```python
from build123d import *
from build123d.topology import SkipClean

# Parameters (mm, degrees)
SKETCH1_R           = 9.525
BOSS_EXTRUDE1_DEPTH = 250
BOSS_EXTRUDE2_DEPTH = 1.5875
CUT_EXTRUDE1_REACH  = 503.261
SKETCH3_R           = 4
SKETCH4_R           = 9.525
BOSS_EXTRUDE3_DEPTH = 50


with BuildPart() as part:
    # Sketch1 → Boss-Extrude1 (new, symmetric)
    with BuildSketch(Plane.XY):
        Circle(SKETCH1_R)
    extrude(amount=BOSS_EXTRUDE1_DEPTH, both=True)

    # Sketch2 → Boss-Extrude2 (add, symmetric)
    with SkipClean():  # the faces are left unmerged after this step: merging them gives an invalid solid
        with BuildSketch(Plane(origin=(0, 0, -250), x_dir=(-1, 0, 0), z_dir=(0, 0, -1))):
            with BuildLine():
                Line((-9.32999835, 1.91748684), (-18.518650577, -42.792134274))
                ThreePointArc((-18.518650577, -42.792134274), (-17.291604236, -47.791622716), (-12.641486262, -50))
                Line((-12.641486262, -50), (12.641486262, -50))
                ThreePointArc((12.641486262, -50), (17.291604236, -47.791622716), (18.518650577, -42.792134274))
                Line((18.518650577, -42.792134274), (9.32999835, 1.91748684))
                ThreePointArc((9.32999835, 1.91748684), (0, 9.525), (-9.32999835, 1.91748684))
            make_face()
        extrude(amount=BOSS_EXTRUDE2_DEPTH, both=True)
    add(part.part.scale(1), mode=Mode.REPLACE)  # the faces are merged on a copy

    # Sketch3 → Cut-Extrude1 (cut, up to next)
    with BuildSketch(Plane.XY.offset(-248.4125), mode=Mode.PRIVATE) as cut_extrude1_sk1:
        with Locations((-12.641486262, -44)):
            Circle(SKETCH3_R)
    cut_extrude1_tool1 = extrude(cut_extrude1_sk1.sketch, amount=-CUT_EXTRUDE1_REACH, mode=Mode.PRIVATE) & part.part
    # Sketch3 → Cut-Extrude1 (cut, up to next)
    with BuildSketch(Plane.XY.offset(-248.4125), mode=Mode.PRIVATE) as cut_extrude1_sk2:
        with Locations((12.641486262, -44)):
            Circle(SKETCH3_R)
    cut_extrude1_tool2 = extrude(cut_extrude1_sk2.sketch, amount=-CUT_EXTRUDE1_REACH, mode=Mode.PRIVATE) & part.part
    add(cut_extrude1_tool1.solids().sort_by_distance((-12.641486, -44, -248.4125))[0], mode=Mode.SUBTRACT)
    add(cut_extrude1_tool2.solids().sort_by_distance((12.641486, -44, -248.4125))[0], mode=Mode.SUBTRACT)

    # Sketch4 → Boss-Extrude3 (add)
    with BuildSketch(Plane(origin=(0, 0, -251.5875), x_dir=(-1, 0, 0), z_dir=(0, 0, -1))):
        Circle(SKETCH4_R)
    extrude(amount=BOSS_EXTRUDE3_DEPTH)


solid = part.part
```
Build history of the part. All positions in model axes, mm. Round coordinates to 2 decimals unless told otherwise and drop trailing zeros. Write each loop counter-clockwise with the first axis right and the second up, starting at its lowest first coordinate (ties: lowest second). Pieces come first, ordered by that corner, then holes. Notation, with made-up numbers: (-13, -8) - (-8, -8) arc R25 cw to (-8, 11) - close; hole circle Ø1 at (65, -7). An arc over 180 degrees is marked (long way). Write each question's results on one line, items separated by ' | '. Start each with the question number.
Item 1: Saw through at B-B (z = 54). Write the cut outline in (x, y) (3 decimals).
Item 2: Saw through at C-C (y = -32.5). Write the cut outline in (x, z).
Item 3: Saw through at A-A (x = 0). Write the cut outline in (y, z) (1 decimal), and give its area (3 significant figures).
Item 4: Drop flat-ended pins along their axis: P1, Ø4, axis at x = -6.5, z = 75.5, coming from the -Y side (3 decimals); P2, Ø1.5, axis at x = -6, y = -28.5, coming from the +Z side; P3, Ø10, axis at x = -6.5, z = -207, coming from the -Y side; P4, Ø6, axis at x = 1, z = -28, coming from the +Y side (3 decimals). Give the stop position or say it passes through.
Item 5: Wall check: L1, parallel to Z at x = -13.5, y = -20.5; L2, parallel to Y at x = 4, z = -41; L3, parallel to X at y = 2, z = -156. Give the ranges that are in metal, low to high. Write a range as [from, to].
Results are:
1) outline: circle Ø19.05 at (0, 0)
2) outline: (-16.4, -251.59) - (16.4, -251.59) - (16.4, -248.41) - (-16.4, -248.41) - close
3) outline: (-50, -251.6) - (-9.5, -251.6) - (-9.5, -301.6) - (9.5, -301.6) - (9.5, 250) - (-9.5, 250) - (-9.5, -248.4) - (-50, -248.4) - close | area: 10,600 mm²
4) P1: stops at y = -8.395 | P2: stops at z = -248.41 | P3: stops at y = -9.41 | P4: stops at y = 9.525
5) L1: z = [-251.59, -248.41] | L2: y = [-8.64, 8.64] | L3: x = [-9.31, 9.31]
